Can you work these out from the model? Positions are in its coordinate system, mm. Give positions to 0.01 mm unless a question says otherwise; leave off trailing zeros. Write each loop counter-clockwise with the first axis right and the second up, starting at its lowest first coordinate (ties: lowest second). Pieces come first, ordered by that corner, then holes. Notation, with made-up numbers: M 1,-28 L 51,-28 A12 cw 51,-17 Z; hole C 1.25,-17 d5. An arc over 180 degrees is marked long. Write each question's results on one line, items separated by ' | '.
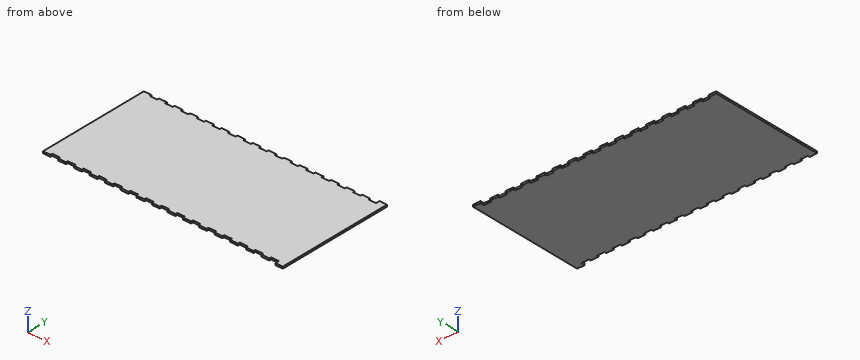
from build123d import *

# Parameters (mm, degrees)
BOSS_EXTRUDE1_DEPTH = 3.175


with BuildPart() as part:
    # Sketch1 → Boss-Extrude1 (new body)
    with BuildSketch(Plane.XY):
        Polygon((-12.6, 186.8186), (-25.5, 186.8186), (-25.5, 190.0936), (-38.907142857, 190.0936), (-38.907142857, 186.8186), (-51.807142857, 186.8186), (-51.807142857, 190.0936), (-65.214285714, 190.0936), (-65.214285714, 186.8186), (-78.114285714, 186.8186), (-78.114285714, 190.0936), (-91.521428571, 190.0936), (-91.521428571, 186.8186), (-104.421428571, 186.8186), (-104.421428571, 190.0936), (-117.828571429, 190.0936), (-117.828571429, 186.8186), (-130.728571429, 186.8186), (-130.728571429, 190.0936), (-144.135714286, 190.0936), (-144.135714286, 186.8186), (-157.035714286, 186.8186), (-157.035714286, 190.0936), (-170.442857143, 190.0936), (-170.442857143, 186.8186), (-183.342857143, 186.8186), (-183.342857143, 190.0936), (-196.75, 190.0936), (-196.75, 186.8186), (-209.65, 186.8186), (-209.65, 190.0936), (-223.057142857, 190.0936), (-223.057142857, 186.8186), (-235.957142857, 186.8186), (-235.957142857, 190.0936), (-249.364285714, 190.0936), (-249.364285714, 186.8186), (-262.264285714, 186.8186), (-262.264285714, 190.0936), (-275.671428571, 190.0936), (-275.671428571, 186.8186), (-288.571428571, 186.8186), (-288.571428571, 190.0936), (-301.978571429, 190.0936), (-301.978571429, 186.8186), (-314.878571429, 186.8186), (-314.878571429, 190.0936), (-328.285714286, 190.0936), (-328.285714286, 186.8186), (-341.185714286, 186.8186), (-341.185714286, 190.0936), (-354.592857143, 190.0936), (-354.592857143, 186.8186), (-367.492857143, 186.8186), (-367.492857143, 190.0936), (-380.9, 190.0936), (-380.9, 186.8186), (-393.8, 186.8186), (-393.8, 190.0936), (-406.4, 190.0936), (-406.4, 0), (-393.8, 0), (-393.8, 3.275), (-380.9, 3.275), (-380.9, 0), (-367.492857143, 0), (-367.492857143, 3.275), (-354.592857143, 3.275), (-354.592857143, 0), (-341.185714286, 0), (-341.185714286, 3.275), (-328.285714286, 3.275), (-328.285714286, 0), (-314.878571429, 0), (-314.878571429, 3.275), (-301.978571429, 3.275), (-301.978571429, 0), (-288.571428571, 0), (-288.571428571, 3.275), (-275.671428571, 3.275), (-275.671428571, 0), (-262.264285714, 0), (-262.264285714, 3.275), (-249.364285714, 3.275), (-249.364285714, 0), (-235.957142857, 0), (-235.957142857, 3.275), (-223.057142857, 3.275), (-223.057142857, 0), (-209.65, 0), (-209.65, 3.275), (-196.75, 3.275), (-196.75, 0), (-183.342857143, 0), (-183.342857143, 3.275), (-170.442857143, 3.275), (-170.442857143, 0), (-157.035714286, 0), (-157.035714286, 3.275), (-144.135714286, 3.275), (-144.135714286, 0), (-130.728571429, 0), (-130.728571429, 3.275), (-117.828571429, 3.275), (-117.828571429, 0), (-104.421428571, 0), (-104.421428571, 3.275), (-91.521428571, 3.275), (-91.521428571, 0), (-78.114285714, 0), (-78.114285714, 3.275), (-65.214285714, 3.275), (-65.214285714, 0), (-51.807142857, 0), (-51.807142857, 3.275), (-38.907142857, 3.275), (-38.907142857, 0), (-25.5, 0), (-25.5, 3.275), (-12.6, 3.275), (-12.6000002, -3.175), (0, -3.175), (0, 193.2686), (-12.6000002, 193.2686), align=None)
    extrude(amount=BOSS_EXTRUDE1_DEPTH)


solid = part.part
Item 1: I'm going to push flat-ended pins straight in: pin 1 (1 mm diameter, centred on x = -151, z = 1, fed in from +Y); pin 2 (1 mm diameter, centred on x = -19, z = 1, fed in from -Y) (3 decimals); pin 3 (1 mm diameter, centred on x = -61.5, z = 1.5, fed in from +Y). Where does each tip first touch, or does it pass through?
Geometry says:
pin 1: stops at y = 186.82 | pin 2: stops at y = 3.275 | pin 3: stops at y = 190.09
Item 2: I want a section at B-B, the plane x = -362. Please give me the cut outline in (y, z) (3 decimals).
Geometry says:
outline: M 3.275,0 L 186.819,0 L 186.819,3.175 L 3.275,3.175 Z
Item 3: I want a section at A-A, the plane x = -60. Please give me the cut outline in (y, z) (3 decimals).
Geometry says:
outline: M 0,0 L 190.094,0 L 190.094,3.175 L 0,3.175 Z
Item 4: If I drill on line 1 (Y direction, x = -360, z = 2.75) (3 decimals); line 2 (Y direction, x = -90.5, z = 3), over which ranges is the centre line in solid material (lowest first)? Write a range as from..to.
Geometry says:
line 1: y = 3.275..186.819 | line 2: y = 0..190.09
